Autodesk Inventor part; units mm, degrees
ref_plane "YZ Plane" through (0, 0, 0) normal (1, 0, 0) x (0, 1, 0)
ref_plane "XZ Plane" through (0, 0, 0) normal (0, 1, 0) x (-1, 0, 0)
ref_plane "XY Plane" through (0, 0, 0) normal (0, 0, 1) x (1, 0, 0)
sketch "Sketch1" plane through (0, 0, 0) normal (0, 1, 0) x (-1, 0, 0)
  line L0 (-11.05, -7.3) -> (11.05, -7.3)
  line L1 (11.05, -7.3) -> (11.05, 7.3)
  line L2 (11.05, 7.3) -> (-11.05, 7.3)
  line L3 (-11.05, 7.3) -> (-11.05, -7.3)
  line L4 (-11.05, -7.3) -> (11.05, 7.3) construction
  line L5 (11.05, -7.3) -> (-11.05, 7.3) construction
  line L6 (0, 3.6568) -> (0, -4.6339)
  line L7 (11.05, 7.3) -> (25, 7.3)
  line L8 (25, 7.3) -> (25, 5.3)
  line L9 (25, 5.3) -> (11.05, 5.3)
  line L10 (11.05, 5.3) -> (11.05, 7.3)
  line L11 (11.05, 7.3) -> (13.05, 7.3)
  line L12 (13.05, 7.3) -> (13.05, -7.3)
  line L13 (13.05, -7.3) -> (11.05, -7.3)
  line L14 (11.05, -7.3) -> (11.05, 7.3)
  line L15 (11.05, 1.3) -> (11.05, 3.3)
  line L16 (11.05, 3.3) -> (13.05, 3.3)
  line L17 (25, 1.3) -> (11.05, 1.3)
  line L18 (25, 3.3) -> (25, 1.3)
  line L19 (11.05, 3.3) -> (25, 3.3)
  line L20 (11.05, -2.7) -> (11.05, -0.7)
  line L21 (11.05, -0.7) -> (13.05, -0.7)
  line L22 (25, -2.7) -> (11.05, -2.7)
  line L23 (25, -0.7) -> (25, -2.7)
  line L24 (11.05, -0.7) -> (25, -0.7)
  line L25 (11.05, -6.7) -> (11.05, -4.7)
  line L26 (11.05, -4.7) -> (13.05, -4.7)
  line L27 (25, -6.7) -> (11.05, -6.7)
  line L28 (25, -4.7) -> (25, -6.7)
  line L29 (11.05, -4.7) -> (25, -4.7)
  point P0 (0, 0)
  dimension "d0" = 22.1
  dimension "d1" = 14.6
  dimension "d2" = 13.95
  dimension "d3" = 2
  dimension "d4" = 2
  dimension "d7" = 4
revolve "Revolution1" add sketch "Sketch1" angle 360 about axis through (0, 0, 3.6568) along (0, 0, -1) contours L1 L27 L12 L13 | L1 L26 L12 L27 | L7 L12 L9 L1 | L1 L22 L12 L26 | L12 L29 L28 L27 | L9 L12 L16 L1 | L7 L8 L9 L12 | L1 L21 L12 L22 | L16 L12 L17 L1 | L1 L17 L12 L21 | L12 L24 L23 L22 | L19 L18 L17 L12
properties part number "HeatSink-H14p6mm"
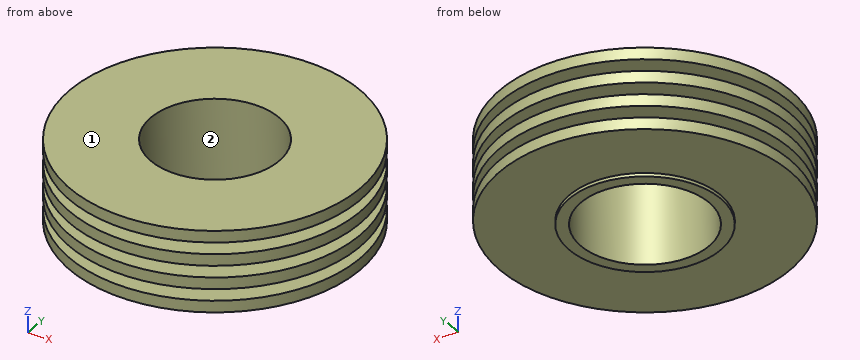
Input: part model. Units: mm. Frame: model coordinates. Face numbers are marked on the shaded views. Coordinates: 2 decimals unless noted, no trailing zeros. Loops run counter-clockwise (first coordinate to the right, second up) from the corner with the lowest first, then second, coordinate; pieces in that order, holes last.
Q1. Mould query, pull axis Y, two halves, no side actions, for the marked faces 1 and 2. Classes: +Y half, -Y half, draft (parallel to the pull), parting line (faces both ways), or undercut.
Results are:
face 1: draft
face 2: undercut
Q2. Section A-A, the plane x = 17. Return the cut outline in (y, z).
Results are:
outline: (-18.33, -6.7) - (18.33, -6.7) - (18.33, -4.7) - (-18.33, -4.7) - close; (-18.33, -2.7) - (18.33, -2.7) - (18.33, -0.7) - (-18.33, -0.7) - close; (-18.33, 1.3) - (18.33, 1.3) - (18.33, 3.3) - (-18.33, 3.3) - close; (-18.33, 5.3) - (18.33, 5.3) - (18.33, 7.3) - (-18.33, 7.3) - close
Q3. Contact query for flat-ended pins moving along their axis: pin 1 (1 mm diameter, centred on x = -6.5, z = 5, fed in from +Y); pin 2 (1 mm diameter, centred on y = 8.5, z = -5, fed in from -X); pin 3 (3 mm diameter, centred on x = -11.5, z = 2.5, fed in from -Y). Output: stop coordinate, or through.
Results are:
pin 1: stops at y = 24.24
pin 2: stops at x = -23.69
pin 3: stops at y = -22.91
Q4. Section C-C, the plane y = -14. Return the cut outline in (x, z).
Results are:
outline: (-20.71, -6.7) - (20.71, -6.7) - (20.71, -4.7) - (-20.71, -4.7) - close; (-20.71, -2.7) - (20.71, -2.7) - (20.71, -0.7) - (-20.71, -0.7) - close; (-20.71, 1.3) - (20.71, 1.3) - (20.71, 3.3) - (-20.71, 3.3) - close; (-20.71, 5.3) - (20.71, 5.3) - (20.71, 7.3) - (-20.71, 7.3) - close
Q5. Line query: line 1 along Z through (x, y) = (-8.5, 20); line 2 along Y through (x, z) = (0, 0.5); line 3 along Y through (x, z) = (0, 2.75). Output: solid intervals per line, ascending.
Results are:
line 1: z = -6.7 to -4.7, -2.7 to -0.7, 1.3 to 3.3, 5.3 to 7.3
line 2: y = -13.05 to -11.05, 11.05 to 13.05
line 3: y = -25 to -11.05, 11.05 to 25
Q6. Section D-D, the plane z = -2. Return the cut outline in (x, y).
Results are:
outline: circle Ø50 at (0, 0); hole circle Ø22.1 at (0, 0)
Q7. Section B-B, the plane z = 4.25. Return the cut outline in (x, y), and give its area (3 significant figures).
Results are:
outline: circle Ø26.1 at (0, 0); hole circle Ø22.1 at (0, 0)
area: 151 mm2
